```python
from build123d import *

# Parameters (mm, degrees)
SKETCH_1_W          = 30
SKETCH_1_H          = 140
EXTRUDE_1_DEPTH     = 10
FILLET_1_RADIUS     = 15
FILLET_1_LENGTH     = 10
CUT_EXTRUDE_1_DEPTH = 10
FILLET_2_R          = 10.407997
SKETCH_3_R          = 2.1
CUT_EXTRUDE_2_DEPTH = 144.527000944
SKETCH_4_R          = 1.35
CUT_EXTRUDE_3_DEPTH = 144.527000944
SKETCH_5_R          = 2.25
EXTRUDE_2_DEPTH     = 35
FILLET_3_R          = 1


with BuildPart() as part:
    # 草图1 → 凸台-拉伸1 (new body)
    with BuildSketch(Plane.XY):
        with Locations((15, 70)):
            Rectangle(SKETCH_1_W, SKETCH_1_H)
    extrude(amount=EXTRUDE_1_DEPTH)

    # 圆角1: full round fillet: the end face becomes a half cylinder, R = half its width
    fillet_1_face = Plane((15, 0, 5), x_dir=(0, 0, 1), z_dir=(0, -1, 0))  # on the end face: x along it, z out of the body
    fillet_1_slab = fillet_1_face.offset(-FILLET_1_RADIUS / 2) * Box(FILLET_1_LENGTH, 2 * FILLET_1_RADIUS, FILLET_1_RADIUS, mode=Mode.PRIVATE)  # the body's end, R deep
    fillet_1_round = Plane((15, 15, 5), x_dir=(0, -1, 0), z_dir=(0, 0, 1)) * Cylinder(FILLET_1_RADIUS, FILLET_1_LENGTH, mode=Mode.PRIVATE)  # its axis R under the face
    add(fillet_1_slab - fillet_1_round, mode=Mode.SUBTRACT)

    # 草图2 → 切除-拉伸1 (cut)
    with BuildSketch(Plane.XY.offset(10)):
        Polygon((0, 15), (5, 140), (0, 140), align=None)
        Polygon((30, 15), (25, 140), (30, 140), align=None)
    extrude(amount=-CUT_EXTRUDE_1_DEPTH, mode=Mode.SUBTRACT)

    # 圆角2
    fillet_2_edges = [part.edges().sort_by_distance(p)[0] for p in [
        (5, 140, 5),
        (25, 140, 5),
    ]]
    fillet(fillet_2_edges, radius=FILLET_2_R - 0.0001)  # a hair under: the kernel refuses the full size

    # 草图3 → 切除-拉伸2 (cut, through all)
    with BuildSketch(Plane.XY.offset(10)):
        with Locations((15, 129.592003197)):
            Circle(SKETCH_3_R)
    extrude(amount=-CUT_EXTRUDE_2_DEPTH, mode=Mode.SUBTRACT)

    # 草图4 → 切除-拉伸3 (cut, through all)
    with BuildSketch(Plane.XY.offset(10)):
        with Locations((15, 8.5)):
            Circle(SKETCH_4_R)
        with Locations((21.5, 15)):
            Circle(SKETCH_4_R)
        with Locations((15, 21.5)):
            Circle(SKETCH_4_R)
        with Locations((8.5, 15)):
            Circle(SKETCH_4_R)
    extrude(amount=-CUT_EXTRUDE_3_DEPTH, mode=Mode.SUBTRACT)

    # 草图5 → 凸台-拉伸2 (add)
    with BuildSketch(Plane.XY.offset(10)):
        with Locations(Location((15, 15, 0), (0, 0, 180))):
            Circle(SKETCH_5_R)
    extrude(amount=EXTRUDE_2_DEPTH)

    # 圆角3
    fillet_3_edges = [part.edges().sort_by_distance(p)[0] for p in [
        (17.25, 15, 10),
    ]]
    fillet(fillet_3_edges, radius=FILLET_3_R)


solid = part.part
```
Verification items for the finished model (mm, model axes). Give positions to 0.01 mm unless a question says otherwise; leave off trailing zeros. Write each loop counter-clockwise with the first axis right and the second up, starting at its lowest first coordinate (ties: lowest second). Pieces come first, ordered by that corner, then holes. Notation, with made-up numbers: (34.5, -37.75) - (76.5, -37.75) arc R27 cw to (76.5, -12.75) - close; hole circle Ø1 at (-32.75, 82.5). An arc over 180 degrees is marked (long way). Put each result on its own line as item: value.
Q1. Scan lines: probe 1 along Y at (x, z) = (15, 6.75); probe 2 along Z at (x, y) = (20.25, 67); probe 3 along Y at (x, z) = (8.5, 5.5). Record each from-to range of solid material in increasing order. Write a range as from..to.
Result:
probe 1: 0..7.15, 9.85..20.15, 22.85..127.49, 131.69..140
probe 2: 0..10
probe 3: 1.48..13.65, 16.35..137.72
Q2. Section check D-D on y = 73. Record the cut outline in (x, z), and give its area (3 significant figures).
Result:
outline: (2.32, 0) - (27.68, 0) - (27.68, 10) - (2.32, 10) - close
area: 254 mm2
Q3. Depth check by flat-ended pin: P1, Ø3.5, axis at x = 8.5, y = 15, coming from the +Z side; P2, Ø1, axis at y = 50, z = 5.5, coming from the +X side; P3, Ø1, axis at y = 45, z = 6, coming from the +X side. Enter the tip coordinate at first touch or a pass-through.
Result:
P1: z = 10
P2: x = 28.62
P3: x = 28.82
Q4. Mould release check, pull along Y, two halves, no side actions. Record for faces 1 (the face through (12.92, 15.86, 27.76)), 2 (the face through (15, 15, 45)), 3 (the face through (27.73, 71.7, 5.07)), 4 (the face through (13.65, 21.56, 5.07)): released by +Y, released by -Y, zero draft, split by the parting line, or undercut.
Result:
face 1: split by the parting line
face 2: zero draft
face 3: released by +Y
face 4: undercut
Q5. Section check C-C on z = 17. Record the cut outline in (x, y).
Result:
outline: circle Ø4.5 at (15, 15)
Q6. Section check A-A on y = 21.5. Record the cut outline in (x, z), and give its area (3 significant figures).
Result:
outline: (0.26, 0) - (13.65, 0) - (13.65, 10) - (0.26, 10) - close; (16.35, 0) - (29.74, 0) - (29.74, 10) - (16.35, 10) - close
area: 268 mm2
Q7. Section check B-B on x = 8.5. Record the cut outline in (y, z), and give its area (3 significant figures).
Result:
outline: (1.48, 0) - (13.65, 0) - (13.65, 10) - (1.48, 10) - close; (16.35, 0) - (137.72, 0) - (137.72, 10) - (16.35, 10) - close
area: 1,340 mm2
